```python
from build123d import *

# Parameters (mm, degrees)
SKETCH1_W           = 20
SKETCH1_H           = 20
SKETCH1_R           = 3.4
BOSS_EXTRUDE1_DEPTH = 25
SKETCH2_W           = 20
SKETCH2_H           = 5
BOSS_EXTRUDE2_DEPTH = 30
SKETCH3_R           = 2.5
CUT_EXTRUDE1_DEPTH  = 58.879184514


with BuildPart() as part:
    # Sketch1 → Boss-Extrude1 (new, symmetric)
    with BuildSketch(Plane(origin=(0, 0, 0), x_dir=(1, 0, 0), z_dir=(0, 1, 0))):
        Rectangle(SKETCH1_W, SKETCH1_H)
        with Locations(Location((0, -0.51, 0), (0, 0, 270))):
            Circle(SKETCH1_R, mode=Mode.SUBTRACT)
    extrude(amount=BOSS_EXTRUDE1_DEPTH, both=True)

    # Sketch2 → Boss-Extrude2 (add)
    with BuildSketch(Plane(origin=(0, 25, 0), x_dir=(1, 0, 0), z_dir=(0, 1, 0))):
        with Locations((0, 7.5)):
            Rectangle(SKETCH2_W, SKETCH2_H)
    extrude(amount=BOSS_EXTRUDE2_DEPTH)

    # Sketch3 → Cut-Extrude1 (cut, through all)
    with BuildSketch(Plane.XY.offset(-5)):
        with Locations((0, 45)):
            Circle(SKETCH3_R)
    extrude(amount=-CUT_EXTRUDE1_DEPTH, mode=Mode.SUBTRACT)


solid = part.part
```
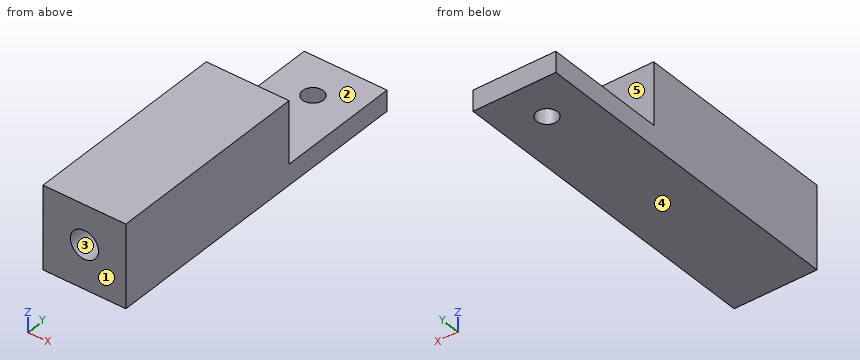
Work out the finished part from the listing and answer in its coordinate system (mm). Face numbers are marked on the shaded views. A direction names the side the tool comes from. Round coordinates to 2 decimals unless told otherwise and drop trailing zeros. Loops run counter-clockwise (first coordinate to the right, second up) from the corner with the lowest first, then second, coordinate; pieces in that order, holes last. Notation, with made-up numbers: (17.5, -21.75) -> (28.5, -21.75) arc R23 ccw to (28.5, 17.25) -> close; hole circle Ø10 at (47.25, 0.25). An arc over 180 degrees is marked (long way). Write each question's results on one line, items separated by ' | '. Start each with the question number.
1. A tool of negligible diameter and unlimited length cuts with its end or side. For the marked faces 1 and 2, from which of +Z, -Z, +X, -X, +Y, -Y can it reach the whole face along a straight path? Write none if from no direction.
2. Given pin 1 Ø9 at (x, z) = (0, 0.51) entering from -Y; pin 2 Ø10 at (x, y) = (-2, 43) entering from +Z; pin 3 Ø7.5 at (x, z) = (4.5, 4.5) entering from +Y, each flat-ended and moving along its own axis, determine where each tip first touches the part or whether it passes through.
3. Find the intervals of material crossed by probe 1 along Y at (x, z) = (0, -8.85); probe 2 along X at (y, z) = (-1.5, 0.51); probe 3 along Z at (x, y) = (-1.75, 28.5), in increasing order. Write a range as from..to.
4. Section C-C (y = 45) is taken. Determine the outline of the cut face in (x, z), plus the area to 3 significant figures.
5. Section B-B (z = 0.51) is taken. Determine the outline of the cut face in (x, y), plus the area to 3 significant figures.
6. For a pull along Z with two mould halves and no side action, classify the marked faces 3, 4 and 5 as +Z half, -Z half, draft (parallel to the pull), parting line (faces both ways), or undercut.
7. Section D-D (y = -1.5) is taken. Determine the outline of the cut face in (x, z).
8. Section A-A (x = 0) is taken. Determine the outline of the cut face in (y, z), plus the area to 3 significant figures.
Evaluation:
1) face 1: +Z, -Z, +X, -X, -Y | face 2: +Z, +X, -X, +Y
2) pin 1: stops at y = -25 | pin 2: stops at z = -5 | pin 3: stops at y = 25
3) probe 1: y = -25..42.5, 47.5..55 | probe 2: x = -10..-3.4, 3.4..10 | probe 3: z = -10..-5
4) outline: (-10, -10) -> (-2.5, -10) -> (-2.5, -5) -> (-10, -5) -> close; (2.5, -10) -> (10, -10) -> (10, -5) -> (2.5, -5) -> close | area: 75.0 mm2
5) outline: (-10, -25) -> (-3.4, -25) -> (-3.4, 25) -> (-10, 25) -> close; (3.4, -25) -> (10, -25) -> (10, 25) -> (3.4, 25) -> close | area: 660 mm2
6) face 3: undercut | face 4: -Z half | face 5: draft
7) outline: (-10, -10) -> (10, -10) -> (10, 10) -> (-10, 10) -> close; hole circle Ø6.8 at (0, 0.51)
8) outline: (-25, -10) -> (42.5, -10) -> (42.5, -5) -> (25, -5) -> (25, -2.89) -> (-25, -2.89) -> close; (-25, 3.91) -> (25, 3.91) -> (25, 10) -> (-25, 10) -> close; (47.5, -10) -> (55, -10) -> (55, -5) -> (47.5, -5) -> close | area: 785 mm2
